Check sheet for the modelled part. Datum: model origin and axes. Units: mm. A direction names the side the tool comes from. Give positions to 0.01 mm unless a question says otherwise; leave off trailing zeros. Answer as CSV lines item,"result". Start each with the question number.
(1) Release check for a two-part mould opening along Y. For faces 5 (the face through (0, 0, 47)), 6 (the face through (229, 0, 1)) record: pulls with the +Y half, pulls with the -Y half, needs draft (parallel to the pull), parting line crosses it, or undercut.
(2) Gauge pin test, flat ends, axial feed: pin 1 Ø1 at (y, z) = (-9, -29.5) entering from +X; pin 2 Ø5 at (x, z) = (30, -19.5) entering from +Y; pin 3 Ø4 at (y, z) = (-42, -10.5) entering from -X. Record the tip position at first contact, or that the pin passes through.
(3) Access from +Z, -Z, +X, -X, +Y, -Y to the whole of each face (thin tool, end or side, straight path). Record for faces 1 (the face through (180, 38, 1)), 2 (the face through (177, 37, -1)), 3 (the face through (300, 0, 47)), 4 (the face through (71, 0, -1)).
(4) Material ranges on line 1 (X direction, y = 43, z = 30); line 2 (Z direction, x = 213, y = 1); line 3 (Z direction, x = 250.5, y = 41), recorded low to high. Write a range as from..to.
from build123d import *

# Parameters (mm, degrees)
SKETCH_1_RX              = 103
SKETCH_1_RY              = 53
SKETCH_1_RX_2            = 96
SKETCH_1_RY_2            = 46
EXTRUDE_1_DEPTH          = 300
SKETCH_2_RX              = 96
SKETCH_2_RY              = 46
EXTRUDE_2_DEPTH          = 30
EXTRUDE_2_DEPTH_BACK     = 30
SKETCH_3_RX              = 96
SKETCH_3_RY              = 46
CUT_EXTRUDE_1_DEPTH      = 27
CUT_EXTRUDE_1_DEPTH_BACK = 27
EXTRUDE_3_DEPTH          = 100
EXTRUDE_4_DEPTH          = 100
EXTRUDE_5_REACH          = 179


with BuildPart() as part:
    # Эскиз1 → Бобышка-Вытянуть1 (new body)
    with BuildSketch(Plane(origin=(0, 0, 0), x_dir=(0, 0, -1), z_dir=(1, 0, 0))):
        with Locations(Location((0, 0), (0, 0, -90))):
            Ellipse(SKETCH_1_RX, SKETCH_1_RY)
        with Locations(Location((0, 0), (0, 0, -90))):
            Ellipse(SKETCH_1_RX_2, SKETCH_1_RY_2, mode=Mode.SUBTRACT)
    extrude(amount=EXTRUDE_1_DEPTH)

    # Эскиз2 → Бобышка-Вытянуть2 (add, two sides)
    with BuildSketch(Plane.ZY.offset(-150)) as extrude_2_sk:
        with Locations(Location((0, 0), (0, 0, -90))):
            Ellipse(SKETCH_2_RX, SKETCH_2_RY)
    extrude(amount=EXTRUDE_2_DEPTH)
    extrude(extrude_2_sk.sketch, amount=-EXTRUDE_2_DEPTH_BACK)

    # Эскиз3 → Вырез-Вытянуть1 (cut, two sides)
    with BuildSketch(Plane.ZY.offset(-150)) as cut_extrude_1_sk:
        with Locations(Location((0, 0), (0, 0, 90))):
            Ellipse(SKETCH_3_RX, SKETCH_3_RY)
    extrude(amount=CUT_EXTRUDE_1_DEPTH, mode=Mode.SUBTRACT)
    extrude(cut_extrude_1_sk.sketch, amount=-CUT_EXTRUDE_1_DEPTH_BACK, mode=Mode.SUBTRACT)

    # Эскиз4 → Бобышка-Вытянуть3 (add)
    with BuildSketch(Plane.ZY.offset(-120)):
        with BuildLine():
            Line((-46, 0), (46, 0))
            add(Edge.make_bspline(
                [(-46, 0), (-46, -96), (0, -96), (46, -96), (46, 0)],
                knots=[4.71238898, 4.71238898, 4.71238898, 6.283185307, 6.283185307, 7.853981634, 7.853981634, 7.853981634], degree=2, weights=[1, 0.707106781, 1, 0.707106781, 1]))
        make_face()
    extrude(amount=EXTRUDE_3_DEPTH)

    # Эскиз5 → Бобышка-Вытянуть4 (add)
    with BuildSketch(Plane(origin=(180, 0, 0), x_dir=(0, 0, -1), z_dir=(1, 0, 0))):
        with BuildLine():
            Line((-46, 0), (46, 0))
            add(Edge.make_bspline(
                [(-46, 0), (-46, -96), (0, -96), (46, -96), (46, 0)],
                knots=[4.71238898, 4.71238898, 4.71238898, 6.283185307, 6.283185307, 7.853981634, 7.853981634, 7.853981634], degree=2, weights=[1, 0.707106781, 1, 0.707106781, 1]))
        make_face()
    extrude(amount=EXTRUDE_4_DEPTH)

    # Эскиз6 → Бобышка-Вытянуть5 (add, up to next)
    with BuildSketch(Plane(origin=(123, 0, 0), x_dir=(0, 0, -1), z_dir=(1, 0, 0)), mode=Mode.PRIVATE) as extrude_5_sk1:
        with BuildLine():
            Line((-46, 0), (46, 0))
            add(Edge.make_bspline(
                [(-46, 0), (-46, -96), (0, -96), (46, -96), (46, 0)],
                knots=[4.71238898, 4.71238898, 4.71238898, 6.283185307, 6.283185307, 7.853981634, 7.853981634, 7.853981634], degree=2, weights=[1, 0.707106781, 1, 0.707106781, 1]))
        make_face()
    extrude_5_tool1 = extrude(extrude_5_sk1.sketch, amount=EXTRUDE_5_REACH, mode=Mode.PRIVATE) - part.part
    add(extrude_5_tool1.solids().sort_by_distance((123, -40.735468, 0))[0])


solid = part.part
Working result:
1,face 5,"needs draft"
1,face 6,"undercut"
2,pin 1,"stops at x = 280"
2,pin 2,"stops at y = 97.56"
2,pin 3,"stops at x = 20"
3,face 1,"+X"
3,face 2,"none"
3,face 3,"+Z, -Z, +X, +Y, -Y"
3,face 4,"-X"
4,line 1,"x = 120..123, 177..180"
4,line 2,"z = -53..-46, 46..53"
4,line 3,"z = -48.62..-41.59, 41.59..48.62"
